The model under review builds one solid part; all positions refer to its coordinate system, in mm. Face numbers are marked on the shaded views. A direction names the side the tool comes from. Round coordinates to 2 decimals unless told otherwise and drop trailing zeros. Write each loop counter-clockwise with the first axis right and the second up, starting at its lowest first coordinate (ties: lowest second). Pieces come first, ordered by that corner, then holes. Notation, with made-up numbers: M -21,85 L -5,85 A19 cw -5,94 Z; hole C 29,7 d10. An arc over 180 degrees is marked long. Write item = value, one per line. Start each with the question number.
Item 1: The part is to be moulded in two halves that separate along Y. For the marked faces 1, 2 and 3, say which applies: +Y half, -Y half, draft (parallel to the pull), parting line (faces both ways), or undercut.
Item 2: Take a section at B-B, the plane x = -6.25. Give the boundary of the cut face in (y, z).
Item 3: For pin 1 Ø6 at (x, y) = (-5.5, 4.5) entering from -Z, flat-tipped, find the tip position at first contact; note if it passes through.
Item 4: Tool access review of the marked faces 4 and 5: name each direction out of +Z, -Z, +X, -X, +Y, -Y from which nothing blocks a thin tool from reaching the whole face with its end or side.
Item 5: Take a section at C-C, the plane z = 2.5. Give the boundary of the cut face in (x, y), plus the area to 3 significant figures.
Item 6: Take a section at A-A, the plane y = 6.5. Give the boundary of the cut face in (x, z), plus the area to 3 significant figures.
Item 7: To check wall thickness, follow line 1 along Y through (x, z) = (6.25, 8.5); line 2 along Y through (x, z) = (6.5, 6.25); line 3 along X through (y, z) = (5.5, 2). State the ranges of each line that lie inside material, in increasing order.
from build123d import *

# Parameters (mm, degrees)
F0_W     = 25
F0_H     = 25
F0_R     = 1.829659
F1_DEPTH = 10


with BuildPart() as f1:
    # F0 (on Top) → F1 (new body)
    with BuildSketch(Plane.XY):
        Rectangle(F0_W, F0_H)
        Polygon((-4.01906, 8.226155), (-3.96133, 5.12945), (-6.61429, 3.531102), (-9.32498, 5.029459), (-9.38271, 8.126164), (-6.72975, 9.724512), align=None, mode=Mode.SUBTRACT)
        with Locations((7.404331, 9.170712)):
            Circle(F0_R, mode=Mode.SUBTRACT)
    extrude(amount=F1_DEPTH)


solid = f1.part
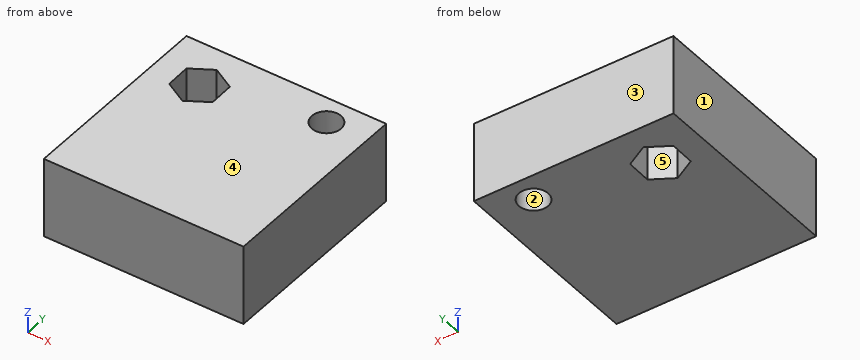
Response values:
q1.face_1 = draft
q1.face_2 = undercut
q1.face_3 = +Y half
q2.outline = M -12.5,0 L 3.75,0 L 3.75,10 L -12.5,10 Z; M 9.46,0 L 12.5,0 L 12.5,10 L 9.46,10 Z
q3.pin_1 = 0
q4.face_4 = +Z, +X, -X, +Y, -Y
q4.face_5 = +Z, -Z
q5.outline = M -12.5,-12.5 L 12.5,-12.5 L 12.5,12.5 L -12.5,12.5 Z; hole M -9.38,8.13 L -9.32,5.03 L -6.61,3.53 L -3.96,5.13 L -4.02,8.23 L -6.73,9.72 Z; hole C 7.4,9.17 d3.66
q5.area = 590 mm2
q6.outline = M -12.5,0 L -9.35,0 L -9.35,10 L -12.5,10 Z; M -3.99,0 L 12.5,0 L 12.5,10 L -3.99,10 Z
q6.area = 196 mm2
q7.line_1 = -12.5 to 7.75, 10.59 to 12.5
q7.line_2 = -12.5 to 7.58, 10.76 to 12.5
q7.line_3 = -12.5 to -9.33, -3.97 to 12.5
